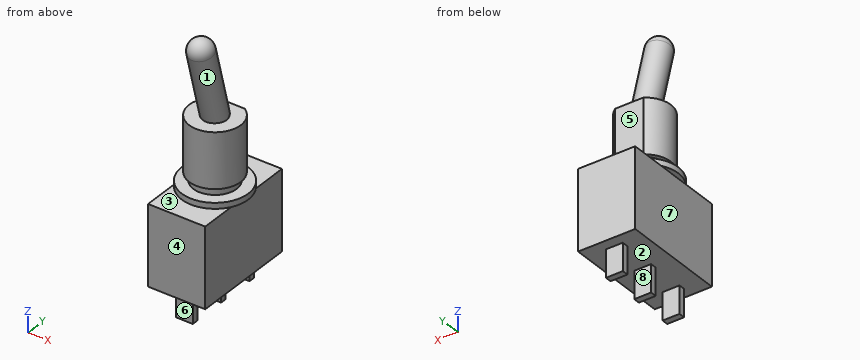
```python
from build123d import *

# Parameters (mm, degrees)
ESQUISSE1_W         = 6.86
ESQUISSE1_H         = 12.7
BOSS_EXTRU_1_DEPTH  = 9.6
SKETCH1_R           = 4
BOSS_EXTRUDE1_DEPTH = 0.7
ESQUISSE4_W         = 2.03
ESQUISSE4_H         = 0.76
BOSS_EXTRU_3_DEPTH  = 3.3
SKETCH3_W           = 6.833076834
SKETCH3_H           = 2.902220806
CUT_EXTRUDE1_DEPTH  = 7.6


with BuildPart() as part:
    # Esquisse1 → Boss.-Extru.1 (new body)
    with BuildSketch(Plane.XY):
        Rectangle(ESQUISSE1_W, ESQUISSE1_H)
    extrude(amount=BOSS_EXTRU_1_DEPTH)

    # Sketch1 → Boss-Extrude1 (add)
    with BuildSketch(Plane(origin=(0, 0, 9.6), x_dir=(-1, 0, 0), z_dir=(0, 0, -1))):
        Circle(SKETCH1_R)
    extrude(amount=-BOSS_EXTRUDE1_DEPTH)

    # Sketch2 → Revolve1 (revolve)
    with BuildSketch(Plane(origin=(0, 0, 0), x_dir=(0, 0, -1), z_dir=(1, 0, 0)), mode=Mode.PRIVATE) as revolve1_sk:
        Polygon((-10.3, 2.6), (-11.3, 2.6), (-11.3, 3.1), (-17.9, 3.1), (-17.9, 0), (-10.3, 0), align=None)
    revolve(revolve1_sk.sketch.rotate(Axis((0, 0, 0), (0, 0, 1)), 90), axis=Axis((0, 0, 0), (0, 0, 1)))

    # Esquisse3 → Révolution1 (revolve)
    with BuildSketch(Plane(origin=(0, 0, 0), x_dir=(0, 0, -1), z_dir=(1, 0, 0))):
        with BuildLine():
            Line((-26.922911951, -0.906178747), (-18.277875806, 1.410251706))
            Line((-18.277875806, 1.410251706), (-17.9, 0))
            Line((-17.9, 0), (-27.955287852, -2.69430626))
            ThreePointArc((-27.955287852, -2.69430626), (-27.809433235, -1.586430454), (-26.922911951, -0.906178747))
        make_face()
    revolve(axis=Axis((0, 0, 17.9), (0, -0.2588190451025217, 0.9659258262890681)))

    # Esquisse4 → Boss.-Extru.3 (add)
    with BuildSketch(Plane.XY):
        Rectangle(ESQUISSE4_W, ESQUISSE4_H)
        with Locations((0, 4.7)):
            Rectangle(ESQUISSE4_W, ESQUISSE4_H)
        with Locations((0, -4.7)):
            Rectangle(ESQUISSE4_W, ESQUISSE4_H)
    extrude(amount=-BOSS_EXTRU_3_DEPTH)

    # Sketch3 → Cut-Extrude1 (cut)
    with BuildSketch(Plane.XY.offset(17.9)):
        with Locations((0.232667491, 4.051110403)):
            Rectangle(SKETCH3_W, SKETCH3_H)
    extrude(amount=-CUT_EXTRUDE1_DEPTH, mode=Mode.SUBTRACT)


solid = part.part
```
Geometry check sheet. Reference: the model listing, model coordinates, mm. Face numbers are marked on the shaded views. A direction names the side the tool comes from. Coordinates: 2 decimals unless noted, no trailing zeros. Order: outer loops, then holes, each group sorted by start corner. A loop starts at its lowest first (then second) coordinate and runs counter-clockwise, first axis right, second up.
Q1. Thickness scan on probe 1 along Z at (x, y) = (-2.25, 0.75); probe 2 along Z at (x, y) = (-2.75, 5.25); probe 3 along X at (y, z) = (1, 7). Record the ranges inside material, lowest first.
Reply:
probe 1: z = 0 to 17.9
probe 2: z = 0 to 9.6
probe 3: x = -3.43 to 3.43
Q2. Sectioned sample at D-D on z = 16.5. Record the cut outline in (x, y).
Reply:
outline: (-1.69, 2.6) arc R3.1 ccw (long way) to (1.69, 2.6) - close
Q3. Sectioned sample at C-C on z = 3. Record the cut outline in (x, y).
Reply:
outline: (-3.43, -6.35) - (3.43, -6.35) - (3.43, 6.35) - (-3.43, 6.35) - close
Q4. Sectioned sample at B-B on z = 11. Record the cut outline in (x, y).
Reply:
outline: circle Ø5.2 at (0, 0)
Q5. Sectioned sample at A-A on x = 2.25. Record the cut outline in (y, z), and give its area (3 significant figures).
Reply:
outline: (-6.35, 0) - (6.35, 0) - (6.35, 9.6) - (3.31, 9.6) - (3.31, 10.3) - (1.3, 10.3) - (1.3, 11.3) - (2.13, 11.3) - (2.13, 17.9) - (-2.13, 17.9) - (-2.13, 11.3) - (-1.3, 11.3) - (-1.3, 10.3) - (-3.31, 10.3) - (-3.31, 9.6) - (-6.35, 9.6) - close
area: 157 mm2
Q6. Depth check by flat-ended pin: pin 1 Ø2 at (x, z) = (0.5, -2) entering from +Y; pin 2 Ø1.3 at (x, y) = (-1.5, 4.5) entering from +Z; pin 3 Ø1 at (x, z) = (0, -1) entering from -Y. Enter the tip coordinate at first touch or a pass-through.
Reply:
pin 1: stops at y = 5.08
pin 2: stops at z = 9.6
pin 3: stops at y = -5.08
Q7. Tool access check on the marked faces 5, 6, 7 and 8. Record the directions out of +Z, -Z, +X, -X, +Y, -Y that give a thin tool (end or side, any length) a straight path to the whole face; none if there is none.
Reply:
face 5: +Z, +X, -X, +Y
face 6: -Z, +X, -X, -Y
face 7: -Z, -X, +Y, -Y
face 8: -Z, +X, -X
Q8. Draft check along Y on the marked faces 1, 2, 3 and 4. Enter one of: released by +Y, released by -Y, zero draft, split by the parting line, or undercut.
Reply:
face 1: split by the parting line
face 2: undercut
face 3: zero draft
face 4: released by -Y
